Build history of the part. All positions in model axes, mm. Face numbers are marked on the shaded views. A direction names the side the tool comes from. Round coordinates to 2 decimals unless told otherwise and drop trailing zeros. Write each loop counter-clockwise with the first axis right and the second up, starting at its lowest first coordinate (ties: lowest second). Pieces come first, ordered by that corner, then holes. Notation, with made-up numbers: (83.5, 11.5) - (118.5, 11.5) arc R26 cw to (118.5, 41.5) - close; hole circle Ø9 at (-4, -7). An arc over 180 degrees is marked (long way). Write each question's results on one line, items separated by ' | '.
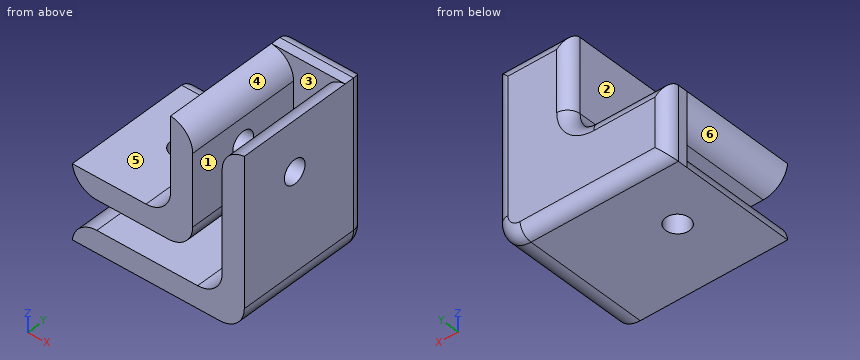
from build123d import *

# Parameters (mm, degrees)
BOSS_EXTRUDE1_DEPTH = 28
CUT_EXTRUDE1_DEPTH  = 23.5
FILLET1_R           = 5
FILLET3_R           = 5
FILLET4_R           = 5
SKETCH3_R           = 2.413
CUT_EXTRUDE2_DEPTH  = 57.868268832
SKETCH4_R           = 2.413
CUT_EXTRUDE3_DEPTH  = 57.868268832
FILLET5_R           = 2.54


with BuildPart() as part:
    # Sketch1 → Boss-Extrude1 (new body)
    with BuildSketch(Plane(origin=(0, 0, 0), x_dir=(1, 0, 0), z_dir=(0, 1, 0))):
        Polygon((0, 0), (-35, 0), (-35, -15), (-15, -15), (-15, -35), (0, -35), align=None)
    extrude(amount=BOSS_EXTRUDE1_DEPTH)

    # Sketch2 → Cut-Extrude1 (cut)
    with BuildSketch(Plane.XZ):
        Polygon((-35, 4.5), (-4.5, 4.5), (-4.5, 35), (-10.5, 35), (-10.5, 10.5), (-35, 10.5), align=None)
    extrude(amount=-CUT_EXTRUDE1_DEPTH, mode=Mode.SUBTRACT)

    # Fillet1
    fillet1_edges = [part.edges().sort_by_distance(p)[0] for p in [
        (-10.5, 11.75, 10.5),
        (-4.5, 11.75, 4.5),
    ]]
    fillet(fillet1_edges, radius=FILLET1_R)

    # Fillet3
    # the kernel refuses this fillet: 5 mm, written as the material it takes off along each edge
    with BuildSketch(Plane(origin=(-4.5, -12.437342964, 35), x_dir=(0, 0, -1), z_dir=(0, 1, 0))) as fillet3_piece_1:
        with BuildLine():
            CenterArc((4.974937186, -5), FILLET3_R, 90, 84.260829523)
            Line((0, -4.5), (0, 0))
            Line((0, 0), (4.974937186, 0))
        make_face()
    extrude(amount=35.937342964, mode=Mode.SUBTRACT)
    with BuildSketch(Plane(origin=(-10.5, -12.437342964, 35), x_dir=(-1, 0, 0), z_dir=(0, 1, 0))) as fillet3_piece_2:
        with BuildLine():
            CenterArc((5, -4.974937186), FILLET3_R, 95.739170477, 84.260829523)
            Line((0, -4.974937186), (0, 0))
            Line((0, 0), (4.5, 0))
        make_face()
    extrude(amount=35.937342964, mode=Mode.SUBTRACT)
    with BuildSketch(Plane(origin=(-35, -12.437342964, 10.5), x_dir=(0, 0, 1), z_dir=(0, 1, 0))) as fillet3_piece_3:
        with BuildLine():
            CenterArc((5, 4.974937186), FILLET3_R, 180, 84.260829523)
            Line((0, 4.974937186), (0, 0))
            Line((0, 0), (4.5, 0))
        make_face()
    extrude(amount=35.937342964, mode=Mode.SUBTRACT)
    with BuildSketch(Plane(origin=(-35, -12.437342964, 4.5), x_dir=(1, 0, 0), z_dir=(0, 1, 0))) as fillet3_piece_4:
        with BuildLine():
            CenterArc((4.974937186, 5), FILLET3_R, 185.739170477, 84.260829523)
            Line((0, 4.5), (0, 0))
            Line((0, 0), (4.974937186, 0))
        make_face()
    extrude(amount=35.937342964, mode=Mode.SUBTRACT)

    # Fillet4
    fillet4_edges = [part.edges().sort_by_distance(p)[0] for p in [
        (-15, 14, 15),
        (0, 14, 0),
    ]]
    fillet(fillet4_edges, radius=FILLET4_R)

    # Sketch3 → Cut-Extrude2 (cut, through all)
    with BuildSketch(Plane(origin=(0, 0, 0), x_dir=(0, 0, -1), z_dir=(1, 0, 0))):
        with Locations((-24.84, 11.75)):
            Circle(SKETCH3_R)
    extrude(amount=-CUT_EXTRUDE2_DEPTH, mode=Mode.SUBTRACT)

    # Sketch4 → Cut-Extrude3 (cut, through all)
    with BuildSketch(Plane(origin=(0, 0, 0), x_dir=(-1, 0, 0), z_dir=(0, 0, -1))):
        with Locations((24.84, 14)):
            Circle(SKETCH4_R)
    extrude(amount=-CUT_EXTRUDE3_DEPTH, mode=Mode.SUBTRACT)

    # Fillet5
    fillet5_edges = [part.edges().sort_by_distance(p)[0] for p in [
        (-20, 28, 0),
        (-15, 28, 27.5),
        (-1.464466094, 28, 1.464466094),
        (-16.464466094, 28, 16.464466094),
        (-35, 28, 7.5),
        (-27.5, 28, 15),
        (-7.5, 28, 35),
        (0, 28, 20),
    ]]
    fillet(fillet5_edges, radius=FILLET5_R)


solid = part.part
(1) Slice it at A-A, the plane z = 24.84. Write the cut outline in (x, y), and give its area (3 significant figures).
Worked answers:
outline: (-15, 0) - (-10.5, 0) - (-10.5, 9.34) - (-15, 9.34) - close; (-15, 14.16) - (-10.5, 14.16) - (-10.5, 23.5) - (-4.5, 23.5) - (-4.5, 14.16) - (0, 14.16) - (0, 25.46) arc R2.54 ccw to (-2.54, 28) - (-12.46, 28) arc R2.54 ccw to (-15, 25.46) - close; (-4.5, 0) - (0, 0) - (0, 9.34) - (-4.5, 9.34) - close | area: 233 mm2
(2) Drill centre lines: probe 1 along Z at (x, y) = (-29.5, 22); probe 2 along X at (y, z) = (16.75, 29); probe 3 along Y at (x, z) = (-11.9, 24.84). Where is each one in solid material? Low to high. Write a range as [from, to].
Worked answers:
probe 1: z = [0, 4.5], [10.5, 15] | probe 2: x = [-15, -10.5], [-4.5, 0] | probe 3: y = [0, 9.34], [14.16, 28]
(3) Two-plate mould, pull along X, no slides. Class the marked faces 4, 5 and 6: released by +X, released by -X, zero draft, split by the parting line, or undercut.
Worked answers:
face 4: undercut | face 5: zero draft | face 6: released by -X
(4) Flat gauge pins, fed straight in: pin 1 Ø6.5 at (y, z) = (11.75, 24.84) entering from -X; pin 2 Ø8 at (y, z) = (12.5, 5.5) entering from -X; pin 3 Ø6 at (x, y) = (-20, 11.5) entering from +Z. Where does each tip first touch, or does it go through?
Worked answers:
pin 1: stops at x = -15 | pin 2: stops at x = -34.61 | pin 3: stops at z = 16
(5) Slice it at C-C, the plane x = -24.84. Write the cut outline in (y, z).
Worked answers:
outline: (0, 0) - (11.59, 0) - (11.59, 4.5) - (0, 4.5) - close; (0, 10.5) - (11.59, 10.5) - (11.59, 15) - (0, 15) - close; (16.41, 0) - (25.46, 0) arc R2.54 ccw to (28, 2.54) - (28, 12.46) arc R2.54 ccw to (25.46, 15) - (16.41, 15) - (16.41, 10.5) - (23.5, 10.5) - (23.5, 4.5) - (16.41, 4.5) - close
(6) Slice it at D-D, the plane y = 10. Write the cut outline in (x, z), and give its area (3 significant figures).
Worked answers:
outline: (-35, 0) - (-5, 0) arc R5 ccw to (0, 5) - (0, 23.18) - (-4.5, 23.18) - (-4.5, 9.5) arc R5 cw to (-9.5, 4.5) - (-30.03, 4.5) arc R5 ccw to start; (-35, 15) arc R5 ccw to (-30.03, 10.5) - (-15.5, 10.5) arc R5 ccw to (-10.5, 15.5) - (-10.5, 23.18) - (-15, 23.18) - (-15, 20) arc R5 cw to (-20, 15) - close; (-15, 26.5) - (-10.5, 26.5) - (-10.5, 30.03) arc R5 ccw to (-15, 35) - close; (-4.5, 26.5) - (0, 26.5) - (0, 35) arc R5 ccw to (-4.5, 30.03) - close | area: 444 mm2
(7) Slice it at B-B, the plane y = 3.75. Write the cut outline in (x, z), and give its area (3 significant figures).
Worked answers:
outline: (-35, 0) - (-5, 0) arc R5 ccw to (0, 5) - (0, 35) arc R5 ccw to (-4.5, 30.03) - (-4.5, 9.5) arc R5 cw to (-9.5, 4.5) - (-30.03, 4.5) arc R5 ccw to start; (-35, 15) arc R5 ccw to (-30.03, 10.5) - (-15.5, 10.5) arc R5 ccw to (-10.5, 15.5) - (-10.5, 30.03) arc R5 ccw to (-15, 35) - (-15, 20) arc R5 cw to (-20, 15) - close | area: 474 mm2
(8) Tool access for the marked faces 1, 2 and 3: list every direction of +Z, -Z, +X, -X, +Y, -Y with a clear straight run to the whole face (end or side of a thin tool).
Worked answers:
face 1: +Z, -Y | face 2: +Z, -X, +Y, -Y | face 3: -Y
